Here's the drawing with two shaded views (mm, measured from the low corner). I have some questions. A direction names the side the tool comes from. Give positions to 0.01 mm unless a question says otherwise; leave off trailing zeros. Loops run counter-clockwise (first coordinate to the right, second up) from the corner with the lowest first, then second, coordinate; pieces in that order, holes last. Notation, with made-up numbers: M -4,16.25 L 19,16.25 A33 ccw 19,50.25 Z; hole C 58,84.5 d2. An arc over 180 degrees is marked long. Put each result on its own line as item: value. Start each with the question number.
1) Imagine slicing it at B-B (y = 12.5). Write out the boundary of the cut face in (x, z).
2) For P1, Ø8, axis at x = 145, y = 12.5, coming from the -Z side; P2, Ø5, axis at x = 71.5, z = 28, coming from the -Y side; P3, Ø3, axis at x = 102.5, z = 30, coming from the +Y side, each with a flat end and sliding along its axis, tell me the tip position at first contact or that it passes through.
3) Imagine slicing it at A-A (x = 145). Write out the boundary of the cut face in (y, z).
4) Please list where these lines run through material, in increasing order: line 1 along Y through (x, z) = (145, 30); line 2 along Z through (x, y) = (75.5, 8.75); line 3 along Y through (x, z) = (70, 26). Write a range as from..to.
5) If we mould it in two halves opening along X, with no side actions, what happens to the marked faces 1, 2 and 3? For each: +X half, -X half, draft (parallel to the pull), parting line (faces both ways), or undercut.
6) Imagine slicing it at D-D (z = 31). Write out the boundary of the cut face in (x, y).
7) Imagine slicing it at C-C (x = 12.5). Write out the boundary of the cut face in (y, z).
8) For the marked faces 4, 5 and 6, which set-ups out of +Z, -Z, +X, -X, +Y, -Y let a thin tool reach every point of the face, with its end or its side?
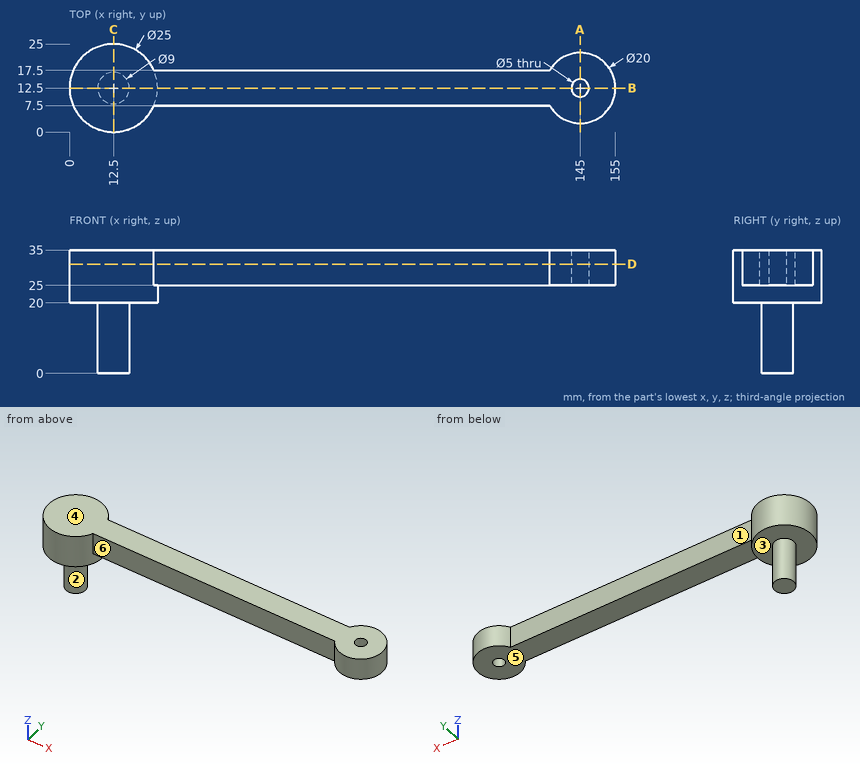
Recorded:
1. outline: M 0,20 L 8,20 L 8,0 L 17,0 L 17,20 L 25,20 L 25,25 L 142.5,25 L 142.5,35 L 0,35 Z; M 147.5,25 L 155,25 L 155,35 L 147.5,35 Z
2. P1: z = 25
2. P2: y = 7.5
2. P3: y = 17.5
3. outline: M 2.5,25 L 10,25 L 10,35 L 2.5,35 Z; M 15,25 L 22.5,25 L 22.5,35 L 15,35 Z
4. line 1: 2.5..10, 15..22.5
4. line 2: 25..35
4. line 3: 7.5..17.5
5. face 1: undercut
5. face 2: parting line
5. face 3: draft
6. outline: M 23.96,7.5 L 136.34,7.5 A10 ccw long 136.34,17.5 L 23.96,17.5 A12.5 ccw long Z; hole C 145,12.5 d5
7. outline: M 0,20 L 8,20 L 8,0 L 17,0 L 17,20 L 25,20 L 25,35 L 0,35 Z
8. face 4: +Z, +X, -X, +Y, -Y
8. face 5: -Z, +X, +Y, -Y
8. face 6: +Z, -Z, -Y
